Model file for the job. Use its own axes, mm. Give positions to 0.01 mm unless a question says otherwise; leave off trailing zeros. Write each loop counter-clockwise with the first axis right and the second up, starting at its lowest first coordinate (ties: lowest second). Pieces come first, ordered by that corner, then holes. Notation, with made-up numbers: (55.5, -1) - (113.5, -1) arc R17 cw to (113.5, 9) - close; hole circle Ø11 at (63, 83.25). An arc over 180 degrees is marked (long way). One line per item, written item: value. Start each with the question number.
(1) Cut at A-A, the plane x = -3.75. List the corners of the cut face in (y, z), and give its area (3 significant figures).
(2) Cut at B-B, the plane z = 9. List the corners of the cut face in (x, y), and give its area (3 significant figures).
(3) Cut at C-C, the plane y = -13. List the corners of the cut face in (x, z), and give its area (3 significant figures).
(4) Drop flat-ended pins along their axis: P1, Ø5, axis at y = -11, z = -11.5, coming from the +X side; P2, Ø4, axis at x = 7.5, y = -11.5, coming from the -Z side; P3, Ø5, axis at x = 8.5, y = -2, coming from the -Z side; P4, Ø13, axis at y = -1.5, z = 0, coming from the -X side. Give the stop position or say it passes through.
(5) Probe L1, parallel to Z at x = 4.5, y = -0.25; L2, parallel to Y at x = -3.5, z = 0. List the from-to ranges inside material, lowest first.
Autodesk Inventor part; units mm, degrees
ref_plane "РабПлоскость1" through (-15, 0, 0) normal (1, 0, 0) x (0, 1, 0)
ref_plane "XZ Plane" through (0, 0, 0) normal (0, 1, 0) x (-1, 0, 0)
ref_plane "XY Plane" through (0, 0, 0) normal (0, 0, 1) x (1, 0, 0)
sketch "Эскиз1" plane through (0, 0, 0) normal (0, 1, 0) x (-1, 0, 0)
  arc A0 (-15, 0) -> (15, 0) centre (0, 0) ccw
  line L0 (15, 0) -> (-15, 0)
  dimension "d0" = 30
revolve "Вращение1" add sketch "Эскиз1" angle 360 about axis through (-15, 0, 0) along (1, 0, 0)
ref_plane "РабПлоскость1" through (-15, 0, 0) normal (1, 0, 0) x (0, 1, 0)
sketch "Эскиз2" plane through (-15, 0, 0) normal (1, 0, 0) x (0, 1, 0)
  point P0 (0, 0)
  point P1 (0, 0)
hole "Отверстие1" at (-15, 0, 0) direction (1, 0, 0) diameter 8.376 depth 22 tip angle 118 counterbore diameter 12 counterbore depth 4
chamfer "Фаска1" distance 1.6 angle 45 1 edges at (-11, 0, -4.188)
properties part number "Ручка-09"
Answers follow:
1. outline: circle Ø29.05 at (0, 0); hole circle Ø8.38 at (0, 0)
1. area: 608 mm²
2. outline: circle Ø24 at (0, 0)
2. area: 452 mm²
3. outline: circle Ø14.97 at (0, 0)
3. area: 176 mm²
4. P1: stops at x = 6.71
4. P2: stops at z = -9.35
4. P3: stops at z = -13.64
4. P4: stops at x = -13.75
5. L1: z = -14.31 to -4.18, 4.18 to 14.31
5. L2: y = -14.59 to -4.19, 4.19 to 14.59
